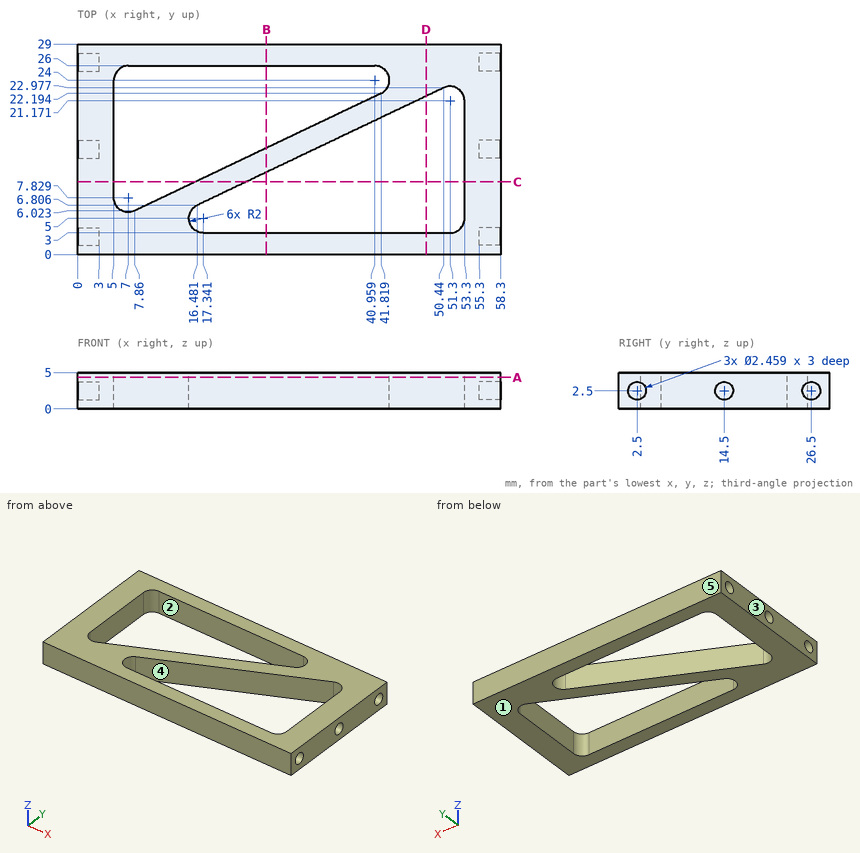
Study the drawing (mm; zero at the part's minimum x, y, z) and answer. A direction names the side the tool comes from. Give positions to 0.01 mm unless a question says otherwise; leave off trailing zeros. Loops run counter-clockwise (first coordinate to the right, second up) from the corner with the lowest first, then second, coordinate; pieces in that order, holes last. Notation, with made-up numbers: (52.25, 50) - (82.25, 50) arc R13 ccw to (82.25, 56) - close; hole circle Ø4 at (19.5, -13). An arc over 180 degrees is marked (long way). Return JSON: item names as keys, results as strings. Group by question number.
1. Straight lines are drawn through the part: line 1 (Y direction, x = 2.25, z = 2.5); line 2 (Z direction, x = 56.6, y = 14.5); line 3 (X direction, y = 10.25, z = 2.7) (1 decimal). For each, find the intervals that lie inside material, in ascending order. Write a range as [from, to].
2. Find section B-B (x = 26). Write down the section's boundary in (y, z), then the cut area to 3 significant figures.
3. Determine the mould class of the marked faces 3, 4 and 5 for opening direction X: pulls with the +X half, pulls with the -X half, needs draft (parallel to the pull), parting line crosses it, or undercut.
4. Find section A-A (z = 4.35). Write down the section's boundary in (x, y).
5. Given pin 1 Ø0.7 at (y, z) = (14.5, 2.5) entering from -X; pin 2 Ø2 at (y, z) = (2.5, 2.5) entering from +X, each flat-ended and moving along its own axis, determine where each tip first touches the part or whether it passes through.
6. Find section C-C (y = 10). Write down the section's boundary in (x, z), then the cut area to 3 significant figures.
7. Find section D-D (x = 48). Write down the section's boundary in (y, z) (1 decimal).
8. Which of the six approach directions +Z, -Z, +X, -X, +Y, -Y give full straight-line access (tool end or side, diameter ignored) to the marked faces 1 and 2?
Verdict:
{
 "1": {"line 1": "y = [0, 1.27], [3.73, 13.27], [15.73, 25.27], [27.73, 29]", "line 2": "z = [0, 1.27], [3.73, 5]", "line 3": "x = [0, 5], [16.7, 23.7], [53.3, 58.3]"},
 "2": {"outline": "(0, 0) - (3, 0) - (3, 5) - (0, 5) - close; (11.34, 0) - (14.66, 0) - (14.66, 5) - (11.34, 5) - close; (26, 0) - (29, 0) - (29, 5) - (26, 5) - close", "area": "46.6 mm^2"},
 "3": {"face 3": "pulls with the -X half", "face 4": "undercut", "face 5": "needs draft"},
 "4": {"outline": "(0, 0) - (58.3, 0) - (58.3, 29) - (0, 29) - close; hole (5, 7.83) arc R2 ccw to (7.86, 6.02) - (41.82, 22.19) arc R2 ccw to (40.96, 26) - (7, 26) arc R2 ccw to (5, 24) - close; hole (16.48, 6.81) arc R2 ccw to (17.34, 3) - (51.3, 3) arc R2 ccw to (53.3, 5) - (53.3, 21.17) arc R2 ccw to (50.44, 22.98) - close"},
 "5": {"pin 1": "stops at x = 3", "pin 2": "stops at x = 55.3"},
 "6": {"outline": "(0, 0) - (5, 0) - (5, 5) - (0, 5) - close; (16.21, 0) - (23.19, 0) - (23.19, 5) - (16.21, 5) - close; (53.3, 0) - (58.3, 0) - (58.3, 5) - (53.3, 5) - close", "area": "84.9 mm^2"},
 "7": {"outline": "(0, 0) - (3, 0) - (3, 5) - (0, 5) - close; (21.8, 0) - (29, 0) - (29, 5) - (21.8, 5) - close"},
 "8": {"face 1": "-Z, +X, -X, +Y, -Y", "face 2": "+Z, -Z"}
}
